Part model, mm, in its own coordinate system. Round coordinates to 2 decimals unless told otherwise and drop trailing zeros. Write each loop counter-clockwise with the first axis right and the second up, starting at its lowest first coordinate (ties: lowest second). Pieces come first, ordered by that corner, then holes. Notation, with made-up numbers: M 84,21.25 L 131,21.25 A27 ccw 131,55.25 Z; hole C 58.25,46.25 d2. An arc over 180 degrees is marked long. Use one line per item in the form item = value. Start each with the question number.
Item 1: Probe L1, parallel to X at y = 45.5, z = 1.3; L2, parallel to X at y = -11, z = 0.7; L3, parallel to Y at x = 42.5, z = 2.3. List the from-to ranges inside material, lowest first.
Item 2: Cut at A-A, the plane x = -38. Give the cut face in (y, z).
Item 3: Mould opens along X. For faces 1 (the face through (-1, 71.5, 1)), 2 (the face through (-45, -16, 1)) say: +X half, -X half, draft (parallel to the pull), parting line (faces both ways), or undercut.
Item 4: Cut at C-C, the plane z = 1.5. State how many separate pieces and enclosed holes the cut face has, then the cut area to 3 significant figures.
Item 5: Cut at D-D, the plane y = 17. Give the cut face in (x, z), then the cut area to 3 significant figures.
Item 6: Cut at B-B, the plane y = -39. Give the cut face in (x, z), then the cut area to 3 significant figures.
from build123d import *

# Parameters (mm, degrees)
F0_W     = 119
F0_H     = 143
F0_W_2   = 13
F0_H_2   = 22
F0_W_3   = 14
F0_W_4   = 18
F0_H_3   = 27
F0_W_5   = 17
F0_W_6   = 23
F0_W_7   = 22
F0_W_8   = 15
F0_W_9   = 21
F1_DEPTH = 3
F2_W     = 1.5
F2_H     = 1
F4_W     = 1.463154
F4_H     = 1.5


with BuildPart() as f1:
    # F0 (on Top) → F1 (new body)
    with BuildSketch(Plane.XY):
        Rectangle(F0_W, F0_H)
        with Locations((-38, -48)):
            Rectangle(F0_W_2, F0_H_2, mode=Mode.SUBTRACT)
        with Locations((-10.5, -48)):
            Rectangle(F0_W_2, F0_H_2, mode=Mode.SUBTRACT)
        with Locations((-38, -16)):
            Rectangle(F0_W_3, F0_H_2, mode=Mode.SUBTRACT)
        with Locations((-10.5, -16)):
            Rectangle(F0_W_2, F0_H_2, mode=Mode.SUBTRACT)
        with Locations((16.07851, -48)):
            Rectangle(F0_W_2, F0_H_2, mode=Mode.SUBTRACT)
        with Locations((41.315013, -48)):
            Rectangle(F0_W_2, F0_H_2, mode=Mode.SUBTRACT)
        with Locations((16.07851, -16)):
            Rectangle(F0_W_2, F0_H_2, mode=Mode.SUBTRACT)
        with Locations((41.315013, -16)):
            Rectangle(F0_W_2, F0_H_2, mode=Mode.SUBTRACT)
        with Locations((-38, 16)):
            Rectangle(F0_W_4, F0_H_3, mode=Mode.SUBTRACT)
        with Locations((-10.5, 16)):
            Rectangle(F0_W_5, F0_H_2, mode=Mode.SUBTRACT)
        with Locations((-38, 48)):
            Rectangle(F0_W_6, F0_H_3, mode=Mode.SUBTRACT)
        with Locations((-10.5, 48)):
            Rectangle(F0_W_7, F0_H_3, mode=Mode.SUBTRACT)
        with Locations((16, 16)):
            Rectangle(F0_W_4, F0_H_3, mode=Mode.SUBTRACT)
        with Locations((40.5, 16)):
            Rectangle(F0_W_8, F0_H_2, mode=Mode.SUBTRACT)
        with Locations((16, 48)):
            Rectangle(F0_W_9, F0_H_3, mode=Mode.SUBTRACT)
        with Locations((40.5, 48)):
            Rectangle(F0_W_4, F0_H_3, mode=Mode.SUBTRACT)
    extrude(amount=F1_DEPTH)

    # F2 (on face) → F3 (revolve)
    with BuildSketch(Plane.XZ.offset(-61.5)):
        with Locations((-37.25, 1.5)):
            Rectangle(F2_W, F2_H)
    revolve(axis=Axis((-38, 61.5, 1.5), (0, 0, -1)))

    # F4 (on face) → F5 (revolve)
    with BuildSketch(Plane.XZ.offset(-61.5)):
        with Locations((-11.231577, 2.25)):
            Rectangle(F4_W, F4_H)
        with Locations((-9.768423, 2.25)):
            Rectangle(F4_W, F4_H)
    revolve(axis=Axis((-10.5, 61.5, 1.5), (-1, 0, 0)))


solid = f1.part
Model answer:
q1.L1 = -59.5 to -49.5, -26.5 to -21.5, 0.5 to 5.5, 26.5 to 31.5, 49.5 to 59.5
q1.L2 = -59.5 to -45, -31 to -17, -4 to 9.58, 22.58 to 34.82, 47.82 to 59.5
q1.L3 = -71.5 to -59, -37 to -27, -5 to 5, 27 to 34.5, 61.5 to 71.5
q2.outline = M -71.5,0 L -59,0 L -59,3 L -71.5,3 Z; M -37,0 L -27,0 L -27,3 L -37,3 Z; M -5,0 L 2.5,0 L 2.5,3 L -5,3 Z; M 29.5,0 L 34.5,0 L 34.5,3 L 29.5,3 Z; M 60,1 L 61.5,1 L 61.5,0 L 71.5,0 L 71.5,3 L 61.5,3 L 61.5,2 L 60,2 Z
q3.face_1 = draft
q3.face_2 = undercut
q4.separate_pieces = 1
q4.enclosed_holes = 16
q4.area = 10,800 mm²
q5.outline = M -59.5,0 L -47,0 L -47,3 L -59.5,3 Z; M -29,0 L -19,0 L -19,3 L -29,3 Z; M -2,0 L 7,0 L 7,3 L -2,3 Z; M 25,0 L 33,0 L 33,3 L 25,3 Z; M 48,0 L 59.5,0 L 59.5,3 L 48,3 Z
q5.area = 153 mm²
q6.outline = M -59.5,0 L -44.5,0 L -44.5,3 L -59.5,3 Z; M -31.5,0 L -17,0 L -17,3 L -31.5,3 Z; M -4,0 L 9.58,0 L 9.58,3 L -4,3 Z; M 22.58,0 L 34.82,0 L 34.82,3 L 22.58,3 Z; M 47.82,0 L 59.5,0 L 59.5,3 L 47.82,3 Z
q6.area = 201 mm²
